Part model, mm, in its own coordinate system. A direction names the side the tool comes from. Coordinates: 2 decimals unless noted, no trailing zeros. Write each loop counter-clockwise with the first axis right and the second up, starting at its lowest first coordinate (ties: lowest second). Pieces come first, ordered by that corner, then holes. Notation, with made-up numbers: (-26.5, 46.5) -> (-3.5, 46.5) arc R24 cw to (-3.5, 68.5) -> close; hole circle Ø2 at (13, 17). An arc over 180 degrees is marked (long way). Write item = value, one per line. Start each with the question number.
Q1. Probe line 1 (X direction, y = 52, z = 9); line 2 (Y direction, x = -49.25, z = 0); line 3 (Z direction, x = 0, y = 40). List the from-to ranges inside material, lowest first.
Q2. Pull direction Z, two halves, no side cores. Call faces 1 (the cylindrical face through (-14.985, 25.35, -0.66)), 2 (the cylindrical face through (47.69, 12.32, -15.02)), 3 (the flat face through (52, 25, 0)): released by +Z, released by -Z, zero draft, split by the parting line, or undercut.
Q3. Tool access for faces 4 (the flat face through (-37.5, 126, 1)), 5 (the cylindrical face through (49.82, 169.83, -2.6)), 6 (the flat face through (-53, 25, -1)): list every direction of +Z, -Z, +X, -X, +Y, -Y with a clear straight run to the whole face (end or side of a thin tool).
Q4. Band-saw the part on B-B, the plane y = 62.5. List the corners of the cut face in (x, z).
Q5. Band-saw the part on C-C, the plane x = -4.5. List the corners of the cut face in (y, z).
Q6. Pin check, flat tips, straight feed: P1, Ø1.5, axis at y = 24.5, z = 5, coming from the -X side; P2, Ø3, axis at x = -4, z = -15, coming from the +Y side; P3, Ø18, axis at x = 0, z = 0, coming from the +Y side. Stop position of each tip, or through.
Q7. Band-saw the part on A-A, the plane z = 0. List the corners of the cut face in (x, y), plus the area to 4 significant figures.
Q8. Band-saw the part on D-D, the plane y = 144. List the corners of the cut face in (x, z).
from build123d import *

# Parameters (mm, degrees)
SKETCH1_R               = 50
SKETCH1_R_2             = 37.5
BOSS_EXTRUDE3_DEPTH     = 25
SKETCH2_R               = 37.5
BOSS_EXTRUDE4_DEPTH     = 25
SKETCH3_W               = 125
SKETCH3_H               = 100
BOSS_EXTRUDE5_DEPTH     = 25
SKETCH4_W               = 25
SKETCH4_H               = 100
BOSS_EXTRUDE6_DEPTH     = 100
SKETCH5_W               = 25
SKETCH5_H               = 100
BOSS_EXTRUDE7_DEPTH     = 100
SKETCH7_R               = 15
CUT_EXTRUDE1_DEPTH      = 101
CUT_EXTRUDE1_DEPTH_BACK = 51
BOSS_EXTRUDE12_DEPTH    = 25
BOSS_EXTRUDE13_DEPTH    = 25
SKETCH14_R              = 20
CUT_EXTRUDE2_DEPTH      = 1
CUT_EXTRUDE2_DEPTH_BACK = 126


with BuildPart() as part:
    # Sketch1 → Boss-Extrude3 (new body)
    with BuildSketch(Plane(origin=(0, 0, 0), x_dir=(1, 0, 0), z_dir=(0, 1, 0))):
        Circle(SKETCH1_R)
        Circle(SKETCH1_R_2, mode=Mode.SUBTRACT)
    extrude(amount=BOSS_EXTRUDE3_DEPTH)

    # Sketch2 → Boss-Extrude4 (add)
    with BuildSketch(Plane.XZ):
        Circle(SKETCH2_R)
    extrude(amount=-BOSS_EXTRUDE4_DEPTH)

    # Sketch3 → Boss-Extrude5 (add)
    with BuildSketch(Plane(origin=(0, 25, 0), x_dir=(1, 0, 0), z_dir=(0, 1, 0))):
        Rectangle(SKETCH3_W, SKETCH3_H)
    extrude(amount=BOSS_EXTRUDE5_DEPTH)

    # Sketch4 → Boss-Extrude6 (add)
    with BuildSketch(Plane(origin=(0, 50, 0), x_dir=(1, 0, 0), z_dir=(0, 1, 0))):
        with Locations((-50, 0)):
            Rectangle(SKETCH4_W, SKETCH4_H)
    extrude(amount=BOSS_EXTRUDE6_DEPTH)

    # Sketch5 → Boss-Extrude7 (add)
    with BuildSketch(Plane(origin=(0, 50, 0), x_dir=(1, 0, 0), z_dir=(0, 1, 0))):
        with Locations((50, 0)):
            Rectangle(SKETCH5_W, SKETCH5_H)
    extrude(amount=BOSS_EXTRUDE7_DEPTH)

    # Sketch7 → Cut-Extrude1 (cut, two sides)
    with BuildSketch(Plane(origin=(0, 50, 0), x_dir=(1, 0, 0), z_dir=(0, 1, 0))) as cut_extrude1_sk:
        Circle(SKETCH7_R)
    extrude(amount=CUT_EXTRUDE1_DEPTH, mode=Mode.SUBTRACT)
    extrude(cut_extrude1_sk.sketch, amount=-CUT_EXTRUDE1_DEPTH_BACK, mode=Mode.SUBTRACT)

    # Sketch11 → Boss-Extrude12 (add)
    with BuildSketch(Plane(origin=(62.5, 0, 0), x_dir=(0, 0, -1), z_dir=(1, 0, 0))):
        with BuildLine():
            Line((-50, 25), (50, 25))
            Line((50, 25), (50, 150))
            ThreePointArc((50, 150), (0, 200), (-50, 150))
            Line((-50, 150), (-50, 25))
        make_face()
    extrude(amount=-BOSS_EXTRUDE12_DEPTH)

    # Sketch13 → Boss-Extrude13 (add)
    with BuildSketch(Plane.ZY.offset(62.5)):
        with BuildLine():
            Line((50, 150), (-50, 150))
            ThreePointArc((-50, 150), (0, 200), (50, 150))
        make_face()
    extrude(amount=-BOSS_EXTRUDE13_DEPTH)

    # Sketch14 → Cut-Extrude2 (cut, two sides)
    with BuildSketch(Plane.ZY.offset(62.5)) as cut_extrude2_sk:
        with Locations((0, 150)):
            Circle(SKETCH14_R)
    extrude(amount=CUT_EXTRUDE2_DEPTH, mode=Mode.SUBTRACT)
    extrude(cut_extrude2_sk.sketch, amount=-CUT_EXTRUDE2_DEPTH_BACK, mode=Mode.SUBTRACT)


solid = part.part
Ans:
q1.line_1 = -62.5 to -37.5, 37.5 to 62.5
q1.line_2 = 0 to 130, 170 to 200
q1.line_3 = -50 to -15, 15 to 50
q2.face_1 = undercut
q2.face_2 = split by the parting line
q2.face_3 = zero draft
q3.face_4 = +Z, -Z, +Y
q3.face_5 = +X, -X
q3.face_6 = -X, -Y
q4.outline = (-62.5, -50) -> (-37.5, -50) -> (-37.5, 50) -> (-62.5, 50) -> close; (37.5, -50) -> (62.5, -50) -> (62.5, 50) -> (37.5, 50) -> close
q5.outline = (0, -49.8) -> (25, -49.8) -> (25, -50) -> (50, -50) -> (50, -14.31) -> (0, -14.31) -> close; (0, 14.31) -> (50, 14.31) -> (50, 50) -> (25, 50) -> (25, 49.8) -> (0, 49.8) -> close
q6.P1 = -62.5
q6.P2 = 50
q6.P3 = through
q7.outline = (-62.5, 25) -> (-50, 25) -> (-50, 0) -> (-15, 0) -> (-15, 50) -> (-37.5, 50) -> (-37.5, 130) -> (-62.5, 130) -> close; (-62.5, 170) -> (-37.5, 170) -> (-37.5, 200) -> (-62.5, 200) -> close; (15, 0) -> (50, 0) -> (50, 25) -> (62.5, 25) -> (62.5, 130) -> (37.5, 130) -> (37.5, 50) -> (15, 50) -> close; (37.5, 170) -> (62.5, 170) -> (62.5, 200) -> (37.5, 200) -> close
q7.area = 9,625 mm2
q8.outline = (-62.5, -50) -> (-37.5, -50) -> (-37.5, -19.08) -> (-62.5, -19.08) -> close; (-62.5, 19.08) -> (-37.5, 19.08) -> (-37.5, 50) -> (-62.5, 50) -> close; (37.5, -50) -> (62.5, -50) -> (62.5, -19.08) -> (37.5, -19.08) -> close; (37.5, 19.08) -> (62.5, 19.08) -> (62.5, 50) -> (37.5, 50) -> close
